from build123d import *

# Parameters (mm, degrees)
F0_W     = 95.25
F0_H     = 95.25
F2_DEPTH = 25.4
F1_R     = 6.399699
F3_DEPTH = 12.7
F4_R     = 3.175
F5_DEPTH = 12.7
F6_R     = 12.7


with BuildPart() as f2:
    # F0 (on Top) → F2 (new body)
    with BuildSketch(Plane.XY):
        Rectangle(F0_W, F0_H)
    extrude(amount=F2_DEPTH)

    # F1 (on Top) → F3 (cut)
    with BuildSketch(Plane.XY):
        with Locations((-31.75, 31.75)):
            Circle(F1_R)
        with Locations((31.75, 31.75)):
            Circle(F1_R)
        with Locations((31.75, -31.75)):
            Circle(F1_R)
        with Locations((-31.75, -31.75)):
            Circle(F1_R)
    extrude(amount=F3_DEPTH, mode=Mode.SUBTRACT)

    # F4 (on face) → F5 (cut)
    with BuildSketch(Plane.XY.offset(25.4)):
        with Locations((-19.05, -19.05)):
            Circle(F4_R)
        with Locations((19.05, -19.05)):
            Circle(F4_R)
        with Locations((19.05, 19.05)):
            Circle(F4_R)
        with Locations((-19.05, 19.05)):
            Circle(F4_R)
    extrude(amount=-F5_DEPTH, mode=Mode.SUBTRACT)

    # F6
    f6_edges = [f2.edges().sort_by_distance(p)[0] for p in [
        (-47.625, 0, 25.4),
        (0, -47.625, 25.4),
        (47.625, 0, 25.4),
        (0, 47.625, 25.4),
    ]]
    fillet(f6_edges, radius=F6_R)


solid = f2.part
Can you work these out from the model? Positions are in its coordinate system, mm. A direction names the side the tool comes from. Give positions to 0.01 mm unless a question says otherwise; leave off trailing zeros. Loops run counter-clockwise (first coordinate to the right, second up) from the corner with the lowest first, then second, coordinate; pieces in that order, holes last. Notation, with made-up numbers: (54, -21) -> (93, -21) arc R29 ccw to (93, 6) -> close; hole circle Ø10 at (46.5, 23.5). An arc over 180 degrees is marked (long way). Return JSON: item names as keys, results as strings.
Q1. For pin 1 Ø4 at (x, y) = (19.05, -19.05) entering from +Z; pin 2 Ø2 at (x, z) = (-27.5, 14) entering from +Y; pin 3 Ø4 at (x, y) = (-29.5, 29.5) entering from -Z, each with a flat end and sliding along its axis, tell me the tip position at first contact or that it passes through.
Checks:
{"pin 1": "stops at z = 12.7", "pin 2": "stops at y = 47.62", "pin 3": "stops at z = 12.7"}
Q2. On a 3-axis mill with a long thin cutter (end or side, diameter ignored), from which of +Z, -Z, +X, -X, +Y, -Y can I reach the whole of each face in a straight line? I mean faces 1 (the face through (-19, -19, 12.7)), 2 (the face through (25.356, 32.031, 6.261)), 3 (the face through (0.667, 44.003, 21.581)). Say none if no direction works.
Checks:
{"face 1": "+Z", "face 2": "-Z", "face 3": "+Z, +X, -X, +Y"}
Q3. I want a section at A-A, the plane x = 19.05. List the corners of the cut face in (y, z) for me (3 decimals), then the cut area to 3 significant figures.
Checks:
{"outline": "(-47.625, 0) -> (47.625, 0) -> (47.625, 12.7) arc R12.7 ccw to (34.925, 25.4) -> (22.225, 25.4) -> (22.225, 12.7) -> (15.875, 12.7) -> (15.875, 25.4) -> (-15.875, 25.4) -> (-15.875, 12.7) -> (-22.225, 12.7) -> (-22.225, 25.4) -> (-34.925, 25.4) arc R12.7 ccw to (-47.625, 12.7) -> close", "area": "2,190 mm2"}
Q4. I need wall thicknesses on probe 1 along Y at (x, z) = (31.75, 5.25) (3 decimals); probe 2 along Y at (x, z) = (-19.05, 19.5) (3 decimals); probe 3 along Z at (x, y) = (17, 20.5). Which ranges of each line are inside material? Lowest first, please.
Checks:
{"probe 1": "y = -47.625 to -38.15, -25.35 to 25.35, 38.15 to 47.625", "probe 2": "y = -45.651 to -22.225, -15.875 to 15.875, 22.225 to 45.651", "probe 3": "z = 0 to 12.7"}
Q5. I want a section at D-D, the plane y = 6.5. List the corners of the cut face in (x, z) for me (3 decimals), then the cut area to 3 significant figures.
Checks:
{"outline": "(-47.625, 0) -> (47.625, 0) -> (47.625, 12.7) arc R12.7 ccw to (34.925, 25.4) -> (-34.925, 25.4) arc R12.7 ccw to (-47.625, 12.7) -> close", "area": "2,350 mm2"}
Q6. I want a section at C-C, the plane z = 22. List the corners of the cut face in (x, y) for me (3 decimals).
Checks:
{"outline": "(-43.574, -43.574) -> (43.574, -43.574) -> (43.574, 43.574) -> (-43.574, 43.574) -> close; hole circle Ø6.35 at (-19.05, -19.05); hole circle Ø6.35 at (-19.05, 19.05); hole circle Ø6.35 at (19.05, -19.05); hole circle Ø6.35 at (19.05, 19.05)"}
Q7. I want a section at B-B, the plane y = 31.75. List the corners of the cut face in (x, z) for me (3 decimals).
Checks:
{"outline": "(-47.625, 0) -> (-38.15, 0) -> (-38.15, 12.7) -> (-25.35, 12.7) -> (-25.35, 0) -> (25.35, 0) -> (25.35, 12.7) -> (38.15, 12.7) -> (38.15, 0) -> (47.625, 0) -> (47.625, 12.7) arc R12.7 ccw to (34.925, 25.4) -> (-34.925, 25.4) arc R12.7 ccw to (-47.625, 12.7) -> close"}
Q8. We'd pull the mould along Y, two halves only. Please class faces 4 (the face through (-19, 19, 12.7)), 5 (the face through (0.667, -44.003, 21.581)), 6 (the face through (47.625, -1, 6)): released by +Y, released by -Y, zero draft, split by the parting line, or undercut.
Checks:
{"face 4": "undercut", "face 5": "released by -Y", "face 6": "zero draft"}
